```python
from build123d import *

# Parameters (mm, degrees)
SKETCH1_R           = 12.5
SKETCH1_R_2         = 8.75
BOSS_EXTRUDE1_DEPTH = 50
BOSS_EXTRUDE2_DEPTH = 50


with BuildPart() as part:
    # Sketch1 → Boss-Extrude1 (new body)
    with BuildSketch(Plane.XY):
        Circle(SKETCH1_R)
        Circle(SKETCH1_R_2, mode=Mode.SUBTRACT)
    extrude(amount=BOSS_EXTRUDE1_DEPTH)

    # Sketch2 → Boss-Extrude2 (add)
    with BuildSketch(Plane.XY):
        with BuildLine():
            Line((-2, -8.518362519), (-2, -2))
            Line((-2, -2), (-8.518362519, -2))
            ThreePointArc((-8.518362519, -2), (-8.75, 0), (-8.518362519, 2))
            Line((-8.518362519, 2), (-2, 2))
            Line((-2, 2), (-2, 8.518362519))
            ThreePointArc((-2, 8.518362519), (0, 8.75), (2, 8.518362519))
            Line((2, 8.518362519), (2, 2))
            Line((2, 2), (8.518362519, 2))
            ThreePointArc((8.518362519, 2), (8.75, 0), (8.518362519, -2))
            Line((8.518362519, -2), (2, -2))
            Line((2, -2), (2, -8.518362519))
            ThreePointArc((2, -8.518362519), (0, -8.75), (-2, -8.518362519))
        make_face()
    extrude(amount=BOSS_EXTRUDE2_DEPTH)


solid = part.part
```
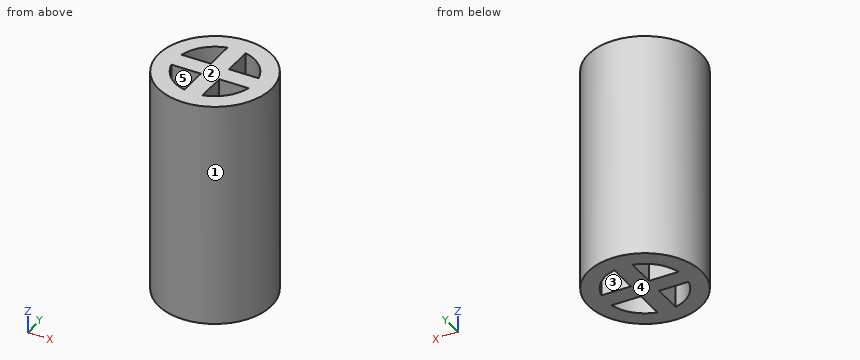
Source: CAD feature listing. Evaluate the final solid. Frame: model axes, mm. Face numbers are marked on the shaded views. A direction names the side the tool comes from. Round coordinates to 2 decimals unless told otherwise and drop trailing zeros. Order: outer loops, then holes, each group sorted by start corner. A loop starts at its lowest first (then second) coordinate and runs counter-clockwise, first axis right, second up. Notation, with made-up numbers: (45.5, 44.5) -> (89.5, 44.5) arc R18 cw to (89.5, 73.5) -> close; hole circle Ø10 at (4.25, -35.75). An arc over 180 degrees is marked (long way). One line per item, written item: value. Start each with the question number.
Q1. Section query B-B (y = -5.75). Return the cut outline in (x, z), plus the area to 3 significant figures.
Q2. Pin query (flat end, axial travel): pin 1 (1 mm diameter, centred on y = 5.5, z = 10.5, fed in from -X); pin 2 (7 mm diameter, centred on y = 4, z = 13.5, fed in from +X); pin 3 (3 mm diameter, centred on x = -6.5, y = 5.5, fed in from +Z); pin 4 (3.5 mm diameter, centred on x = 5.5, z = 14, fed in from -Y). Return the tip coordinate at first contact, or that it passes through.
Q3. Section query A-A (z = 28). Return the cut outline in (x, y), plus the area to 3 significant figures.
Q4. Section query C-C (x = -4.25). Return the cut outline in (y, z).
Q5. Draft query along Y for the marked faces 1, 2 and 3. Return one class per face: pulls with the +Y half, pulls with the -Y half, needs draft (parallel to the pull), parting line crosses it, or undercut.
Q6. Material intervals for probe 1 along Y at (x, z) = (-6.75, 15); probe 2 along X at (y, z) = (3, 29); probe 3 along Y at (x, z) = (-3.75, 42.5), sorted ascending.
Q7. Section query D-D (x = 10). Return the cut outline in (y, z), plus the area to 3 significant figures.
Q8. Access query for the marked faces 4 and 5. Directions: +Z, -Z, +X, -X, +Y, -Y. A direction counts if a zero-diameter tool reaches every point of the face in a straight line with its end or side. Return the directions, or none.
Findings below:
1. outline: (-11.1, 0) -> (-6.6, 0) -> (-6.6, 50) -> (-11.1, 50) -> close; (-2, 0) -> (2, 0) -> (2, 50) -> (-2, 50) -> close; (6.6, 0) -> (11.1, 0) -> (11.1, 50) -> (6.6, 50) -> close
1. area: 650 mm²
2. pin 1: x = -11.46
2. pin 2: x = 12.49
2. pin 3: z = 50
2. pin 4: y = -11.92
3. outline: circle Ø25 at (0, 0); hole (-8.52, -2) arc R8.75 ccw to (-2, -8.52) -> (-2, -2) -> close; hole (-8.52, 2) -> (-2, 2) -> (-2, 8.52) arc R8.75 ccw to start; hole (2, -8.52) arc R8.75 ccw to (8.52, -2) -> (2, -2) -> close; hole (2, 2) -> (8.52, 2) arc R8.75 ccw to (2, 8.52) -> close
3. area: 373 mm²
4. outline: (-11.76, 0) -> (-7.65, 0) -> (-7.65, 50) -> (-11.76, 50) -> close; (-2, 0) -> (2, 0) -> (2, 50) -> (-2, 50) -> close; (7.65, 0) -> (11.76, 0) -> (11.76, 50) -> (7.65, 50) -> close
5. face 1: parting line crosses it
5. face 2: needs draft
5. face 3: undercut
6. probe 1: -10.52 to -5.57, -2 to 2, 5.57 to 10.52
6. probe 2: -12.13 to -8.22, -2 to 2, 8.22 to 12.13
6. probe 3: -11.92 to -7.91, -2 to 2, 7.91 to 11.92
7. outline: (-7.5, 0) -> (7.5, 0) -> (7.5, 50) -> (-7.5, 50) -> close
7. area: 750 mm²
8. face 4: -Z, +X, -X, +Y, -Y
8. face 5: +Z, -Z
